```python
from build123d import *

# Parameters (mm, degrees)
F0_R     = 7.9375
F0_R_2   = 12.7
F0_R_3   = 6.35
F1_DEPTH = 6.35


with BuildPart() as f1:
    # F0 (on Front) → F1 (new body, symmetric)
    with BuildSketch(Plane.XZ):
        with BuildLine():
            ThreePointArc((82.55, -7.463384), (50.109619, 24.279109), (19.080024, -8.843819))
            ThreePointArc((19.080024, -8.843819), (17.762053, -12.344458), (14.322027, -13.813384))
            Line((14.322027, -13.813384), (0, -13.813384))
            Line((0, -13.813384), (-14.322027, -13.813384))
            ThreePointArc((-14.322027, -13.813384), (-17.762053, -12.344458), (-19.080024, -8.843819))
            ThreePointArc((-19.080024, -8.843819), (-50.109619, 24.279109), (-82.55, -7.463384))
            Line((-82.55, -7.463384), (-82.55, -34.931994))
            ThreePointArc((-82.55, -34.931994), (-83.623483, -37.944063), (-86.36, -39.598272))
            ThreePointArc((-86.36, -39.598272), (-101.503534, -60.17808), (-82.55, -77.313384))
            Line((-82.55, -77.313384), (-53.975, -77.313384))
            ThreePointArc((-53.975, -77.313384), (-47.239808, -80.103192), (-44.45, -86.838384))
            Line((-44.45, -86.838384), (-44.45, -93.188384))
            ThreePointArc((-44.45, -93.188384), (-41.660192, -99.923576), (-34.925, -102.713384))
            Line((-34.925, -102.713384), (-19.030211, -102.713384))
            Line((-19.030211, -102.713384), (-19.030211, -90.013384))
            ThreePointArc((-19.030211, -90.013384), (-0.516209, -70.970926), (19.039627, -88.941812))
            Line((19.039627, -88.941812), (19.030211, -102.713384))
            Line((19.030211, -102.713384), (34.925, -102.713384))
            ThreePointArc((34.925, -102.713384), (41.660192, -99.923576), (44.45, -93.188384))
            Line((44.45, -93.188384), (44.45, -86.838384))
            ThreePointArc((44.45, -86.838384), (47.239808, -80.103192), (53.975, -77.313384))
            Line((53.975, -77.313384), (82.55, -77.313384))
            ThreePointArc((82.55, -77.313384), (101.503534, -60.17808), (86.36, -39.598272))
            ThreePointArc((86.36, -39.598272), (83.623483, -37.944063), (82.55, -34.931994))
            Line((82.55, -34.931994), (82.55, -7.463384))
        make_face()
        with Locations((-82.55, -58.263384)):
            Circle(F0_R, mode=Mode.SUBTRACT)
        with Locations((0, -42.388384)):
            Circle(F0_R_2, mode=Mode.SUBTRACT)
        with Locations((82.55, -58.263384)):
            Circle(F0_R, mode=Mode.SUBTRACT)
        with Locations((-50.8, -7.463384)):
            Circle(F0_R_2, mode=Mode.SUBTRACT)
        with Locations((50.8, -7.463384)):
            Circle(F0_R_2, mode=Mode.SUBTRACT)
        with Locations((82.55, -58.263384)):
            Circle(F0_R)
        with Locations((82.55, -58.263384)):
            Circle(F0_R_3, mode=Mode.SUBTRACT)
        with Locations((-82.55, -58.263384)):
            Circle(F0_R)
        with Locations((-82.55, -58.263384)):
            Circle(F0_R_3, mode=Mode.SUBTRACT)
    extrude(amount=F1_DEPTH, both=True)


solid = f1.part
```
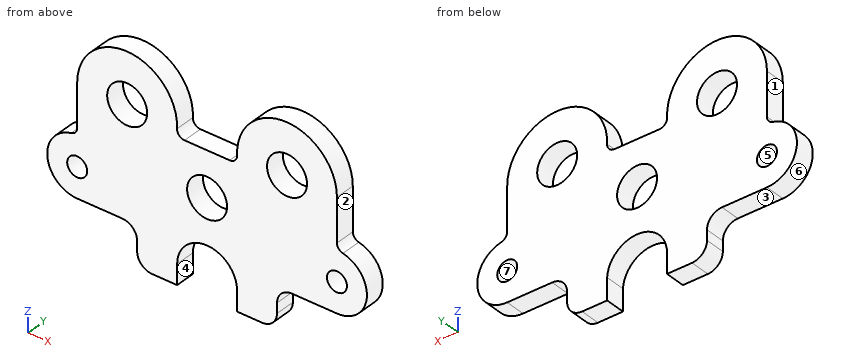
Input: part model. Units: mm. Frame: model coordinates. Face numbers are marked on the shaded views. A direction names the side the tool comes from. Coordinates: 2 decimals unless noted, no trailing zeros. Loops run counter-clockwise (first coordinate to the right, second up) from the corner with the lowest first, then second, coordinate; pieces in that order, holes last. Notation, with made-up numbers: M -30.75,7.5 L -23.75,7.5 A11 cw -23.75,20.5 Z; hole C -10,44 d7. An arc over 180 degrees is marked long. Use a Markdown table: item, result. Add a question column.
1) Set-up query: the marked faces 1, 2 and 3. Return all of +Z, -Z, +X, -X, +Y, -Y with unobstructed straight access to the full face (end or side cutting, diameter ignored); none if empty.
2) Section C-C, the plane y = -1. Give the number of separate pieces and of enclosed holes in the cut face, plus the area to 3 significant figures.
3) Section B-B, the plane z = -48.5. Return the cut outline in (x, y), plus the area to 3 significant figures.
4) Section A-A, the plane x = 0. Return the cut outline in (y, z).
5) Line query: L1, parallel to Z at x = 0, y = 2.25; L2, parallel to X at y = 4.25, z = -59.5; L3, parallel to X at y = -4.75, z = -6.5. Output: solid intervals per line, ascending. Write a range as from..to.
6) Pin query (flat end, axial travel): P1, Ø10, axis at x = -82.55, z = -58.26, coming from the +Y side; P2, Ø7, axis at y = -1, z = -91, coming from the +X side; P3, Ø6, axis at y = 3, z = -75.5, coming from the -X side; P4, Ø5, axis at y = 1, z = -88.5, coming from the -X side. Return the tip coordinate at first contact, or that it passes through.
7) Draft query along Z for the marked faces 4, 5, 6 and 7. Return one class per face: +Z half, -Z half, draft (parallel to the pull), parting line (faces both ways), or undercut.
8) Section D-D, the plane x = -21.5. Return the cut outline in (y, z).
Answer below:
| question | item | result |
|---|---|---|
| 1 | face 1 | +Z, -X, +Y, -Y |
| 1 | face 2 | +Z, +X, +Y, -Y |
| 1 | face 3 | -Z, -X, +Y, -Y |
| 2 | separate pieces | 1 |
| 2 | enclosed holes | 5 |
| 2 | area | 15,000 mm2 |
| 3 | outline | M -98.91,-6.35 L -11.13,-6.35 L -11.13,6.35 L -98.91,6.35 Z; M 11.13,-6.35 L 98.91,-6.35 L 98.91,6.35 L 11.13,6.35 Z |
| 3 | area | 2,230 mm2 |
| 4 | outline | M -6.35,-70.96 L 6.35,-70.96 L 6.35,-55.09 L -6.35,-55.09 Z; M -6.35,-29.69 L 6.35,-29.69 L 6.35,-13.81 L -6.35,-13.81 Z |
| 5 | L1 | -70.96..-55.09, -29.69..-13.81 |
| 5 | L2 | -101.56..-88.78, -76.32..76.32, 88.78..101.56 |
| 5 | L3 | -82.54..-63.46, -38.14..-19.06, 19.06..38.14, 63.46..82.54 |
| 6 | P1 | through |
| 6 | P2 | x = 44.45 |
| 6 | P3 | x = -95.21 |
| 6 | P4 | x = -44.49 |
| 7 | face 4 | draft |
| 7 | face 5 | undercut |
| 7 | face 6 | parting line |
| 7 | face 7 | undercut |
| 8 | outline | M -6.35,-102.71 L 6.35,-102.71 L 6.35,4.77 L -6.35,4.77 Z |
